```python
from build123d import *

# Parameters (mm, degrees)
SKETCH1_R           = 2.05
BOSS_EXTRUDE1_DEPTH = 2.2
THREAD1_PITCH       = 0.6


with BuildPart() as part:
    # Sketch1 → Boss-Extrude1 (new body)
    with BuildSketch(Plane.XY):
        Polygon((-3.464101615, -2), (0, -4), (3.464101615, -2), (3.464101615, 2), (0, 4), (-3.464101615, 2), align=None)
        Circle(SKETCH1_R, mode=Mode.SUBTRACT)
    extrude(amount=BOSS_EXTRUDE1_DEPTH)

    # Thread1: the profile of Thread Profile1 profile screwed along a right-hand helix of 3.666667 turns, 6 arcs to a turn; built about Z, then put on its axis
    thread1_z = Axis((0, 0, 0), (0, 0, 1))
    thread1_corners = [(2.0497, 0, -0.000173205), (2.374759525, 0, 0.187499999), (2.374759525, 0, 0.262499999), (2.0497, 0, 0.450173203)]
    with BuildLine(mode=Mode.PRIVATE) as thread1_profile:
        Line(thread1_corners[0], thread1_corners[1])
        Line(thread1_corners[1], thread1_corners[2])
        Line(thread1_corners[2], thread1_corners[3])
        Line(thread1_corners[3], thread1_corners[0])
    thread1_cap = Face(thread1_profile.wire())
    thread1_turn_angles = [0, 30, 60, 90, 120, 150, 180, 210, 240, 270, 300, 330, 360]
    thread1_turn_weights = [1, 0.8660254037844387, 1, 0.8660254037844387, 1, 0.8660254037844387, 1, 0.8660254037844387, 1, 0.8660254037844387, 1, 0.8660254037844387, 1]
    thread1_turn_rails = [Edge.make_bspline([Vector(p[0], p[1], 0).rotate(thread1_z, thread1_turn_angles[k]) / thread1_turn_weights[k] + Vector(0, 0, p[2] + THREAD1_PITCH * thread1_turn_angles[k] / 360) for k in range(13)], [0, 0, 0, 1, 1, 2, 2, 3, 3, 4, 4, 5, 5, 6, 6, 6], 2, thread1_turn_weights) for p in thread1_corners]
    thread1_turn_sides = [Face.make_surface_from_curves(thread1_turn_rails[p[0]], thread1_turn_rails[p[1]]) for p in [(0, 1), (1, 2), (2, 3), (3, 0)]]
    thread1_last_angles = [1080, 1110, 1140, 1170, 1200, 1230, 1260, 1290, 1320]
    thread1_last_weights = [1, 0.8660254037844387, 1, 0.8660254037844387, 1, 0.8660254037844387, 1, 0.8660254037844377, 1]
    thread1_last_rails = [Edge.make_bspline([Vector(p[0], p[1], 0).rotate(thread1_z, thread1_last_angles[k]) / thread1_last_weights[k] + Vector(0, 0, p[2] + THREAD1_PITCH * thread1_last_angles[k] / 360) for k in range(9)], [0, 0, 0, 1, 1, 2, 2, 3, 3, 4, 4, 4], 2, thread1_last_weights) for p in thread1_corners]
    thread1_last_sides = [Face.make_surface_from_curves(thread1_last_rails[p[0]], thread1_last_rails[p[1]]) for p in [(0, 1), (1, 2), (2, 3), (3, 0)]]
    thread1 = Plane(origin=(0, 0, 2.2), x_dir=(-1, 0, 0), z_dir=(0, 0, -1)) * Solid(Shell([*[p.moved(Location((0, 0, THREAD1_PITCH * i))) for i in range(3) for p in thread1_turn_sides], *thread1_last_sides, thread1_cap, thread1_cap.rotate(thread1_z, 1320).moved(Location((0, 0, THREAD1_PITCH * 1320 / 360)))]))
    add(thread1, mode=Mode.SUBTRACT)


solid = part.part
```
For this review, take the finished solid that the model builds, in its own axes (mm). Round coordinates to 2 decimals unless told otherwise and drop trailing zeros. Order: outer loops, then holes, each group sorted by start corner. A loop starts at its lowest first (then second) coordinate and runs counter-clockwise, first axis right, second up. Notation, with made-up numbers: (48, 13.25) -> (77, 13.25) arc R33 ccw to (77, 52.25) -> close; hole circle Ø11 at (17.25, -10). An arc over 180 degrees is marked (long way). Use a Markdown table: item, result.
Item 1: For line 1 along Z through (x, y) = (-0.5, 2.25); line 2 along X through (y, z) = (0, 0.6); line 3 along Z through (x, y) = (2, -1), list the stretches that pass through material, from the lowest coordinate up. Write a range as [from, to].
Resolved:
| item | result |
|---|---|
| line 1 | z = [0.12, 0.57], [0.72, 1.17], [1.32, 1.77], [1.92, 2.2] |
| line 2 | x = [-3.46, -2.14], [2.22, 3.46] |
| line 3 | z = [0, 0.31], [0.55, 0.91], [1.15, 1.51], [1.75, 2.2] |
Item 2: Take a section at A-A (y = 3.75). State the section outline as (x, z) points.
Resolved:
| item | result |
|---|---|
| outline | (-0.43, 0) -> (0.43, 0) -> (0.43, 2.2) -> (-0.43, 2.2) -> close |
Item 3: Take a section at B-B (x = -2.5). State the section outline as (y, z) points, plus the area to 3 significant figures.
Resolved:
| item | result |
|---|---|
| outline | (-2.56, 0) -> (2.56, 0) -> (2.56, 2.2) -> (-2.56, 2.2) -> close |
| area | 11.2 mm² |
Item 4: For pin 1 (3 mm diameter, centred on x = 0.5, y = 2.5, fed in from -Z), flat-tipped, find the tip position at first contact; note if it passes through.
Resolved:
| item | result |
|---|---|
| pin 1 | stops at z = 0 |
